Work out the finished part from the listing and answer in its coordinate system (mm). Face numbers are marked on the shaded views. A direction names the side the tool comes from. Round coordinates to 2 decimals unless told otherwise and drop trailing zeros. Loops run counter-clockwise (first coordinate to the right, second up) from the corner with the lowest first, then second, coordinate; pieces in that order, holes last. Notation, with made-up numbers: (26.25, 39) - (40.25, 39) arc R34 ccw to (40.25, 70) - close; hole circle Ø9 at (58, -18). An arc over 180 degrees is marked (long way). Use CSV: the item, a comma, the result in double quotes. Start each with the question number.
from build123d import *

# Parameters (mm, degrees)
CROQUIS2_W              = 43
CROQUIS2_H              = 30
SALIENTE_EXTRUIR1_DEPTH = 30
CROQUIS3_W              = 42.529407755
CROQUIS3_H              = 25.558495791
CORTAR_EXTRUIR1_DEPTH   = 30
CORTAR_EXTRUIR2_START   = -7.5
CORTAR_EXTRUIR2_DEPTH   = 15
CORTAR_EXTRUIR4_DEPTH   = 4.5
CORTAR_EXTRUIR5_DEPTH   = 4.5
REDONDEO1_R             = 3
CROQUIS8_W              = 15
CROQUIS8_H              = 32.397186909
CORTAR_EXTRUIR6_DEPTH   = 4.5
CROQUIS9_W              = 120.283196461
CROQUIS9_H              = 78.810135234
CORTAR_EXTRUIR7_DEPTH   = 22.5
CORTAR_EXTRUIR8_DEPTH   = 22.5


with BuildPart() as part:
    # Croquis2 → Saliente-Extruir1 (new body)
    with BuildSketch(Plane(origin=(0, 0, 0), x_dir=(0, 0, -1), z_dir=(1, 0, 0))):
        with Locations((-19.783269962, -13.522813688)):
            Rectangle(CROQUIS2_W, CROQUIS2_H)
    extrude(amount=SALIENTE_EXTRUIR1_DEPTH)

    # Croquis3 → Cortar-Extruir1 (cut)
    with BuildSketch(Plane(origin=(30, 0, 0), x_dir=(0, 0, -1), z_dir=(1, 0, 0))):
        with Locations((-17.018566085, -31.302061584)):
            Rectangle(CROQUIS3_W, CROQUIS3_H)
        Polygon((-31.675073764, 1.477186312), (-3.283269962, -16.522813688), (1.716730038, -16.522813688), (1.716730038, 1.477186312), align=None)
    extrude(amount=-CORTAR_EXTRUIR1_DEPTH, mode=Mode.SUBTRACT)

    # Croquis4 → Cortar-Extruir2 (cut)
    with BuildSketch(Plane(origin=(30, 0, 0), x_dir=(0, 0, -1), z_dir=(1, 0, 0)).offset(CORTAR_EXTRUIR2_START)):
        Polygon((-41.283269962, -1.522813688), (-32.545919554, -1.522813688), (-8.886083053, -16.522813688), (-41.283269962, -16.522813688), align=None)
    extrude(amount=-CORTAR_EXTRUIR2_DEPTH, mode=Mode.SUBTRACT)

    # Croquis5 → Cortar-Extruir4 (cut)
    with BuildSketch(Plane(origin=(30, 0, 0), x_dir=(0, 0, -1), z_dir=(1, 0, 0))):
        Polygon((-3.283269962, -16.522813688), (-41.283269962, -16.522813688), (-41.283269962, 1.477186312), (-31.675073764, 1.477186312), align=None)
    extrude(amount=-CORTAR_EXTRUIR4_DEPTH, mode=Mode.SUBTRACT)

    # Croquis6 → Cortar-Extruir5 (cut)
    with BuildSketch(Plane.ZY):
        Polygon((3.283269962, -16.522813688), (41.283269962, -16.522813688), (41.283269962, 1.477186312), (31.675073764, 1.477186312), align=None)
    extrude(amount=-CORTAR_EXTRUIR5_DEPTH, mode=Mode.SUBTRACT)

    # Redondeo1
    redondeo1_edges = [part.edges().sort_by_distance(p)[0] for p in [
        (0, -17.522813688, -1.716730038),
        (30, -17.522813688, -1.716730038),
    ]]
    fillet(redondeo1_edges, radius=REDONDEO1_R)

    # Croquis8 → Cortar-Extruir6 (cut)
    with BuildSketch(Plane(origin=(0, -16.522813688, 0), x_dir=(1, 0, 0), z_dir=(0, 1, 0))):
        with Locations((15, -25.084676508)):
            Rectangle(CROQUIS8_W, CROQUIS8_H)
    extrude(amount=-CORTAR_EXTRUIR6_DEPTH, mode=Mode.SUBTRACT)

    # Croquis9 → Cortar-Extruir7 (cut)
    with BuildSketch(Plane.XZ.offset(18.522813688)):
        with Locations((17.6156444, 62.089659259)):
            Rectangle(CROQUIS9_W, CROQUIS9_H)
    extrude(amount=CORTAR_EXTRUIR7_DEPTH, mode=Mode.SUBTRACT)

    # Croquis10 → Cortar-Extruir8 (cut)
    with BuildSketch(Plane(origin=(25.5, 0, 0), x_dir=(0, 0, -1), z_dir=(1, 0, 0))):
        Polygon((-41.283269962, -1.522813688), (-32.545919554, -1.522813688), (-8.886083053, -16.522813688), (1.716730038, -16.522813688), (-27.710183608, 4.902177411), (-44.228495628, 5.2702735), align=None)
    extrude(amount=-CORTAR_EXTRUIR8_DEPTH, mode=Mode.SUBTRACT)


solid = part.part
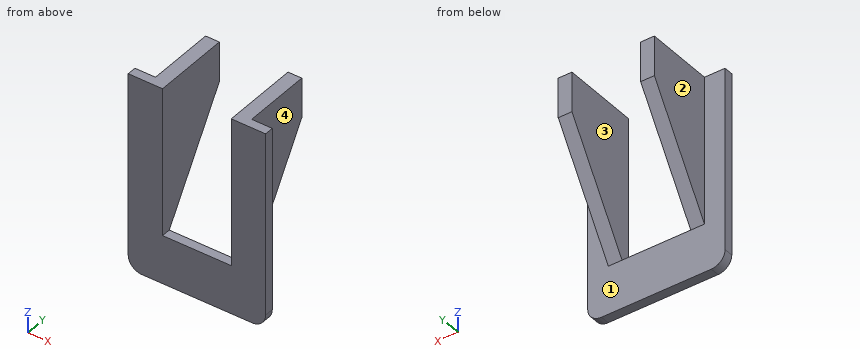
Item 1: Find the intervals of material crossed by probe 1 along X at (y, z) = (-12.75, 25); probe 2 along X at (y, z) = (-17.5, 19); probe 3 along Y at (x, z) = (28, 14.5), in increasing order. Write a range as [from, to].
Item 2: Each of these flat-tipped pins is pushed along its axis until it touches: pin 1 Ø4.5 at (y, z) = (-5.5, 21.5) entering from -X; pin 2 Ø5 at (y, z) = (-12.5, 19) entering from -X; pin 3 Ø8 at (x, z) = (23.5, 31) entering from +Y; pin 4 Ø1.6 at (x, y) = (16.5, -18) entering from +Z. Where does it stop, or does it pass through?
Item 3: A cutting plane is placed at A-A (z = 33.5). Determine the outline of the cut face in (x, y).
Item 4: A cutting plane is placed at D-D (y = -9.5). Determine the outline of the cut face in (x, z), plus the area to 3 significant figures.
Item 5: A cutting plane is placed at B-B (y = -4.5). Determine the outline of the cut face in (x, z), plus the area to 3 significant figures.
Item 6: Which of the six approach directions +Z, -Z, +X, -X, +Y, -Y give full straight-line access (tool end or side, diameter ignored) to the marked faces 1, 2, 3 and 4?
Item 7: A cutting plane is placed at C-C (z = 10). Determine the outline of the cut face in (x, y), plus the area to 3 significant figures.
Result sheet:
1,probe 1,"[4.5, 7.5], [22.5, 25.5]"
1,probe 2,"[0, 7.5], [22.5, 30]"
1,probe 3,"[-18.52, -16.52]"
2,pin 1,"through"
2,pin 2,"x = 4.5"
2,pin 3,"y = -1.52"
2,pin 4,"z = 8.89"
3,outline,"(0, -18.52) - (7.5, -18.52) - (7.5, -1.52) - (4.5, -1.52) - (4.5, -16.52) - (0, -16.52) - close; (22.5, -18.52) - (30, -18.52) - (30, -16.52) - (25.5, -16.52) - (25.5, -1.52) - (22.5, -1.52) - close"
4,outline,"(4.5, 19.96) - (7.5, 19.96) - (7.5, 41.28) - (4.5, 41.28) - close; (22.5, 19.96) - (25.5, 19.96) - (25.5, 41.28) - (22.5, 41.28) - close"
4,area,"128 mm^2"
5,outline,"(4.5, 27.85) - (7.5, 27.85) - (7.5, 41.28) - (4.5, 41.28) - close; (22.5, 27.85) - (25.5, 27.85) - (25.5, 41.28) - (22.5, 41.28) - close"
5,area,"80.6 mm^2"
6,face 1,"-Z, +Y"
6,face 2,"+Z, -Z, -X, +Y"
6,face 3,"+Z, +Y, -Y"
6,face 4,"+Z, -Z, +X, +Y"
7,outline,"(0, -18.52) - (7.5, -18.52) - (7.5, -15.82) - (4.5, -15.82) - (4.5, -16.52) - (0, -16.52) - close; (22.5, -18.52) - (30, -18.52) - (30, -16.52) - (25.5, -16.52) - (25.5, -15.82) - (22.5, -15.82) - close"
7,area,"34.2 mm^2"
